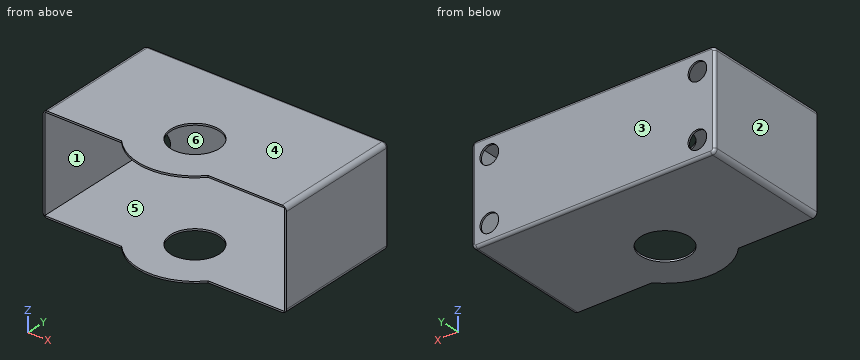
from build123d import *

# Parameters (mm, degrees)
BOSS_EXTRU_1_DEPTH      = 55
COQUE1_T                = -2
ESQUISSE2_R             = 27.5
ENL_V_MAT_EXTRU_1_DEPTH = 200.841186946
ESQUISSE3_R             = 10.5
ENL_V_MAT_EXTRU_2_DEPTH = 224.204502643
CONG_2_R                = 3
CONG_3_R                = 5


with BuildPart() as part:
    # Esquisse1 → Boss.-Extru.1 (new, symmetric)
    with BuildSketch(Plane.XY):
        with BuildLine():
            Line((-137.5, 72.5), (137.5, 72.5))
            Line((137.5, 72.5), (137.5, -72.5))
            Line((137.5, -72.5), (48.744230428, -72.5))
            ThreePointArc((48.744230428, -72.5), (0, -94.5), (-48.744230428, -72.5))
            Line((-48.744230428, -72.5), (-137.5, -72.5))
            Line((-137.5, -72.5), (-137.5, 72.5))
        make_face()
    extrude(amount=BOSS_EXTRU_1_DEPTH, both=True)

    # Coque1
    coque1_openings = [part.faces().sort_by_distance(p)[0] for p in [
        (93.122115214, -72.5, 0),
        (0, -94.5, 0),
        (-93.122115214, -72.5, 0),
    ]]
    offset(amount=COQUE1_T, openings=coque1_openings, kind=Kind.INTERSECTION)

    # Esquisse2 → Enlèv. mat.-Extru.1 (cut, through all)
    with BuildSketch(Plane(origin=(0, 0, -55), x_dir=(-1, 0, 0), z_dir=(0, 0, -1))):
        with Locations((0, -29.5)):
            Circle(ESQUISSE2_R)
    extrude(amount=-ENL_V_MAT_EXTRU_1_DEPTH, mode=Mode.SUBTRACT)

    # Esquisse3 → Enlèv. mat.-Extru.2 (cut, through all)
    with BuildSketch(Plane(origin=(0, 72.5, 0), x_dir=(1, 0, 0), z_dir=(0, 1, 0))):
        with Locations(Location((-117.5, 35, 0), (0, 0, 270))):
            Circle(ESQUISSE3_R)
        with Locations(Location((-117.5, -35, 0), (0, 0, 270))):
            Circle(ESQUISSE3_R)
        with Locations(Location((117.5, 35, 0), (0, 0, 90))):
            Circle(ESQUISSE3_R)
        with Locations(Location((117.5, -35, 0), (0, 0, 90))):
            Circle(ESQUISSE3_R)
    extrude(amount=-ENL_V_MAT_EXTRU_2_DEPTH, mode=Mode.SUBTRACT)

    # Congé2
    cong_2_edges = [part.edges().sort_by_distance(p)[0] for p in [
        (-137.5, 72.5, 0),
        (137.5, 72.5, 0),
        (0, 72.5, 55),
        (0, 72.5, -55),
    ]]
    fillet(cong_2_edges, radius=CONG_2_R)

    # Congé3
    # the kernel refuses this fillet: 5 mm, written as the material it takes off along each edge
    with BuildSketch(Plane(origin=(-132.5, 72.5, 50), x_dir=(-1, 0, 0), z_dir=(0, 0, -1))) as cong_3_piece_1:
        with BuildLine():
            CenterArc((2, -3), 3, 0, 90)
            Line((5, -3), (5, 0))
            Line((5, 0), (2, 0))
        make_face()
    revolve(axis=Axis((-132.5, 72.5, 50), (0, 1, 0)), revolution_arc=90, mode=Mode.SUBTRACT)
    with BuildSketch(Plane(origin=(-132.5, 72.5, -50), x_dir=(0, 0, -1), z_dir=(1, 0, 0))) as cong_3_piece_2:
        with BuildLine():
            CenterArc((2, -3), 3, 0, 90)
            Line((5, -3), (5, 0))
            Line((5, 0), (2, 0))
        make_face()
    revolve(axis=Axis((-132.5, 72.5, -50), (0, 1, 0)), revolution_arc=90, mode=Mode.SUBTRACT)
    with BuildSketch(Plane(origin=(132.5, 72.5, 50), x_dir=(0, 0, 1), z_dir=(-1, 0, 0))) as cong_3_piece_3:
        with BuildLine():
            CenterArc((2, -3), 3, 0, 90)
            Line((5, -3), (5, 0))
            Line((5, 0), (2, 0))
        make_face()
    revolve(axis=Axis((132.5, 72.5, 50), (0, 1, 0)), revolution_arc=90, mode=Mode.SUBTRACT)
    with BuildSketch(Plane(origin=(132.5, 72.5, -50), x_dir=(1, 0, 0), z_dir=(0, 0, 1))) as cong_3_piece_4:
        with BuildLine():
            CenterArc((2, -3), 3, 0, 90)
            Line((5, -3), (5, 0))
            Line((5, 0), (2, 0))
        make_face()
    revolve(axis=Axis((132.5, 72.5, -50), (0, 1, 0)), revolution_arc=90, mode=Mode.SUBTRACT)
    with BuildSketch(Plane(origin=(137.5, 72.5, 55), x_dir=(-1, 0, 0), z_dir=(0, -1, 0)), Plane(origin=(137.5, 72.5, -55), x_dir=(0, 0, 1), z_dir=(0, -1, 0)), Plane(origin=(-137.5, -85, -55), x_dir=(0, 0, 1), z_dir=(0, 1, 0)), Plane(origin=(-137.5, -85, 55), x_dir=(1, 0, 0), z_dir=(0, 1, 0))) as cong_3_piece_5:
        with BuildLine():
            CenterArc((CONG_3_R, CONG_3_R), CONG_3_R, 180, 90)
            Line((0, CONG_3_R), (0, 0))
            Line((0, 0), (CONG_3_R, 0))
        make_face()
    extrude(amount=157.5, mode=Mode.SUBTRACT)


solid = part.part
The model under review builds one solid part; all positions refer to its coordinate system, in mm. Face numbers are marked on the shaded views. A direction names the side the tool comes from. Round coordinates to 2 decimals unless told otherwise and drop trailing zeros. Order: outer loops, then holes, each group sorted by start corner. A loop starts at its lowest first (then second) coordinate and runs counter-clockwise, first axis right, second up. Notation, with made-up numbers: (85.25, -31) -> (126.25, -31) arc R17 cw to (126.25, -22) -> close; hole circle Ø11 at (29.25, 30.25). An arc over 180 degrees is marked (long way). Write item = value, one per line. Start each with the question number.
Item 1: Consider section C-C on z = -35. Write out the cut boundary in (x, y), plus the area to 3 significant figures.
Item 2: Consider section A-A on y = -13. Write out the cut boundary in (x, z).
Item 3: Clearance check with flat-ended pins moving along their axes: pin 1 Ø8 at (x, z) = (98.5, -17) entering from -Y; pin 2 Ø17 at (x, z) = (117.5, 35) entering from +Y. State where each tip first meets the part, or that it passes through.
Item 4: For line 1 along Z through (x, y) = (79.5, 8); line 2 along X through (y, z) = (53, -28.5); line 3 along X through (y, z) = (71, 35), list the stretches that pass through material, from the lowest coordinate up.
Item 5: Consider section B-B on x = -117.5. Write out the cut boundary in (y, z).
Item 6: Consider section D-D on y = 4. Write out the cut boundary in (x, z), plus the area to 3 significant figures.
Item 7: Mouldability with a two-part tool opening along Z and no side actions: class the marked faces 3, 4, 5 and 6 as released by +Z, released by -Z, zero draft, split by the parting line, or undercut.
Item 8: For the marked faces 1 and 2, list the 3-axis set-ups (+Z, -Z, +X, -X, +Y, -Y) from which the entire face can be reached by the end or side of a thin tool; tool diameter is ignored.
Conclusion:
q1.outline = (-137.5, -72.5) -> (-135.5, -72.5) -> (-135.5, 70.5) -> (-128, 70.5) -> (-128, 72.5) -> (-134.5, 72.5) arc R3 ccw to (-137.5, 69.5) -> close; (-107, 70.5) -> (107, 70.5) -> (107, 72.5) -> (-107, 72.5) -> close; (128, 70.5) -> (135.5, 70.5) -> (135.5, -72.5) -> (137.5, -72.5) -> (137.5, 69.5) arc R3 ccw to (134.5, 72.5) -> (128, 72.5) -> close
q1.area = 1,030 mm2
q2.outline = (-137.5, -50) arc R5 ccw to (-132.5, -55) -> (-22, -55) -> (-22, -53) -> (-135.5, -53) -> (-135.5, 53) -> (-22, 53) -> (-22, 55) -> (-132.5, 55) arc R5 ccw to (-137.5, 50) -> close; (22, -55) -> (132.5, -55) arc R5 ccw to (137.5, -50) -> (137.5, 50) arc R5 ccw to (132.5, 55) -> (22, 55) -> (22, 53) -> (135.5, 53) -> (135.5, -53) -> (22, -53) -> close
q3.pin_1 = 70.5
q3.pin_2 = through
q4.line_1 = -55 to -53, 53 to 55
q4.line_2 = -137.5 to -135.5, 135.5 to 137.5
q4.line_3 = -137.1 to -128, -107 to 107, 128 to 137.1
q5.outline = (-72.5, -55) -> (69.5, -55) arc R3 ccw to (72.5, -52) -> (72.5, -45.5) -> (70.5, -45.5) -> (70.5, -53) -> (-72.5, -53) -> close; (-72.5, 53) -> (70.5, 53) -> (70.5, 45.5) -> (72.5, 45.5) -> (72.5, 52) arc R3 ccw to (69.5, 55) -> (-72.5, 55) -> close; (70.5, -24.5) -> (72.5, -24.5) -> (72.5, 24.5) -> (70.5, 24.5) -> close
q6.outline = (-137.5, -50) arc R5 ccw to (-132.5, -55) -> (132.5, -55) arc R5 ccw to (137.5, -50) -> (137.5, 50) arc R5 ccw to (132.5, 55) -> (-132.5, 55) arc R5 ccw to (-137.5, 50) -> close; hole (-135.5, -53) -> (135.5, -53) -> (135.5, 53) -> (-135.5, 53) -> close
q6.area = 1,500 mm2
q7.face_3 = zero draft
q7.face_4 = released by +Z
q7.face_5 = undercut
q7.face_6 = undercut
q8.face_1 = -Y
q8.face_2 = +Z, -Z, -X, +Y, -Y
